from build123d import *

# Parameters (mm, degrees)
BOSS_EXTRUDE1_DEPTH = 31.75
SKETCH3_R           = 4.7625
SKETCH3_R_2         = 1.6383
CUT_EXTRUDE1_DEPTH  = 47.337599474
SKETCH4_R           = 1.524
CUT_EXTRUDE2_DEPTH  = 47.337599474


with BuildPart() as part:
    # Sketch2 → Boss-Extrude1 (new body)
    with BuildSketch(Plane(origin=(0, 0, 0), x_dir=(0, 0, -1), z_dir=(1, 0, 0))):
        Polygon((0, 0), (25.4, 0), (25.4, 3.175), (3.175, 3.175), (3.175, 25.4), (0, 25.4), align=None)
    extrude(amount=BOSS_EXTRUDE1_DEPTH)

    # Sketch3 → Cut-Extrude1 (cut, through all)
    with BuildSketch(Plane(origin=(0, 0, -3.175), x_dir=(-1, 0, 0), z_dir=(0, 0, -1))):
        with Locations((-15.875, 19.05)):
            Circle(SKETCH3_R)
        with Locations((-7.366, 19.05)):
            Circle(SKETCH3_R_2)
        with Locations((-24.384, 19.05)):
            Circle(SKETCH3_R_2)
    extrude(amount=-CUT_EXTRUDE1_DEPTH, mode=Mode.SUBTRACT)

    # Sketch4 → Cut-Extrude2 (cut, through all)
    with BuildSketch(Plane(origin=(0, 3.175, 0), x_dir=(1, 0, 0), z_dir=(0, 1, 0))):
        with Locations(Location((5.08, 21.59, 0), (0, 0, 270))):
            Circle(SKETCH4_R)
        with Locations(Location((26.67, 10.16, 0), (0, 0, 270))):
            Circle(SKETCH4_R)
    extrude(amount=-CUT_EXTRUDE2_DEPTH, mode=Mode.SUBTRACT)


solid = part.part
CAD build for the part. Positions are in the model's coordinates, mm. A direction names the side the tool comes from. Give positions to 0.01 mm unless a question says otherwise; leave off trailing zeros. Loops run counter-clockwise (first coordinate to the right, second up) from the corner with the lowest first, then second, coordinate; pieces in that order, holes last. Notation, with made-up numbers: M 65.25,72 L 116.25,72 A22 ccw 116.25,108 Z; hole C 58.25,1.5 d5. An arc over 180 degrees is marked long. One line per question, with ' | ' between items. Start each with the question number.
1. Saw through at D-D on y = 16.5. Give the cut face in (x, z) (3 decimals).
2. Saw through at B-B on x = 5.08. Give the cut face in (y, z) (3 decimals), plus the area to 3 significant figures.
3. Saw through at C-C on y = 19.05. State how many separate pieces and enclosed holes the cut face has, plus the area to 3 significant figures.
4. Probe L1, parallel to X at y = 0.8, z = -21.59; L2, parallel to Y at x = 4.5, z = -13.5 (3 decimals); L3, parallel to Z at x = 21.5, y = 3.5 (3 decimals). List the from-to ranges inside material, lowest first. Write a range as from..to.
5. 3-axis set-ups, long thin cutter, end or side, ignore diameter. For faces 4 (the face through (16, 14, -3.175)), 5 (the face through (7.72, 17.45, -1.61)): which of +Z, -Z, +X, -X, +Y, -Y reach the whole face in a straight line?
6. Saw through at A-A on z = -21.59. Give the cut face in (x, y) (3 decimals), plus the area to 3 significant figures.
7. Flat gauge pins, fed straight in: pin 1 (2.5 mm diameter, centred on x = 7.366, y = 19.05, fed in from -Z); pin 2 (12.5 mm diameter, centred on x = 15.875, y = 19.05, fed in from -Z) (3 decimals). Where does each tip first touch, or does it go through?
8. Two-plate mould, pull along Y, no slides. Class faces 1 (the face through (16, 0, -13)), 2 (the face through (19.385, 22.269, -1.61)), 3 (the face through (16, 25.4, -2)): pulls with the +Y half, pulls with the -Y half, needs draft (parallel to the pull), parting line crosses it, or undercut.
Result sheet:
1) outline: M 0,-3.175 L 11.853,-3.175 L 11.853,0 L 0,0 Z; M 19.897,-3.175 L 31.75,-3.175 L 31.75,0 L 19.897,0 Z
2) outline: M 0,-25.4 L 3.175,-25.4 L 3.175,-23.114 L 0,-23.114 Z; M 0,-20.066 L 3.175,-20.066 L 3.175,-3.175 L 25.4,-3.175 L 25.4,0 L 0,0 Z | area: 142 mm^2
3) separate pieces: 4 | enclosed holes: 0 | area: 49.8 mm^2
4) L1: x = 0..3.56, 6.6..31.75 | L2: y = 0..3.175 | L3: z = -3.175..0
5) face 4: -Z, +X, -X, +Y | face 5: +Z, -Z
6) outline: M 0,0 L 3.556,0 L 3.556,3.175 L 0,3.175 Z; M 6.604,0 L 31.75,0 L 31.75,3.175 L 6.604,3.175 Z | area: 91.1 mm^2
7) pin 1: passes through | pin 2: stops at z = -3.175
8) face 1: pulls with the -Y half | face 2: undercut | face 3: pulls with the +Y half
